Input: part model. Units: mm. Frame: model coordinates. Coordinates: 2 decimals unless noted, no trailing zeros. Write each loop counter-clockwise with the first axis right and the second up, starting at its lowest first coordinate (ties: lowest second). Pieces come first, ordered by that corner, then holes. Notation, with made-up numbers: (40, 19.25) -> (52, 19.25) arc R27 ccw to (52, 43.25) -> close; hole circle Ø2 at (89, 51.25). An arc over 180 degrees is marked (long way). Use one line per item in the form item = value. Start each with the question number.
(1) Cut plane D-D on x = 15.5. Return the cut outline in (y, z), plus the area to 3 significant figures.
(2) Ray query, line 1 along Z through (x, y) = (-4, 0.9); line 2 along Z through (x, y) = (0, 0.5); line 3 along X through (y, z) = (1, 1.75). Return the intervals inside material, ascending.
(3) Cut plane A-A on y = 1. State how many separate pieces and enclosed holes the cut face has, plus the area to 3 significant figures.
(4) First-contact query: pin 1 (4 mm diameter, centred on x = 16, z = 1.5, fed in from -Y). Flat tip, straight axial feed; report the tip coordinate or a pass-through.
(5) Cut plane C-C on x = -8. Return the cut outline in (y, z), plus the area to 3 significant figures.
(6) Cut plane B-B on x = 3. Return the cut outline in (y, z), plus the area to 3 significant figures.
Autodesk Inventor part; units mm, degrees
ref_plane "YZ Plane" through (0, 0, 0) normal (1, 0, 0) x (0, 1, 0)
ref_plane "XZ Plane" through (0, 0, 0) normal (0, 1, 0) x (-1, 0, 0)
ref_plane "XY Plane" through (0, 0, 0) normal (0, 0, 1) x (1, 0, 0)
sketch "Sketch2" plane through (0, 0, 0) normal (0, 1, 0) x (-1, 0, 0)
  line L0 (-32, 4) -> (32, 4)
  line L1 (32, 4) -> (32, -4)
  line L2 (32, -4) -> (-32, -4)
  line L3 (-32, -4) -> (-32, 4)
  point P0 (0, 0)
  point P1 (0, 4)
  point P2 (-32, 0)
  dimension "d0" = 64
  dimension "d1" = 8
extrude "Extrusion1" add sketch "Sketch2" along normal blind 3.2
sketch "Sketch3" plane through (0, 0, 0) normal (0, -1, 0) x (1, 0, 0)
  line L0 (32, 4) -> (-32, 4)
  line L1 (-32, 4) -> (-32, -4)
  line L2 (-30.4, 2.4) -> (30.4, 2.4)
  line L3 (30.4, 2.4) -> (30.4, -2.4)
  line L4 (30.4, -2.4) -> (-30.4, -2.4)
  line L5 (-30.4, -2.4) -> (-30.4, 2.4)
  circle A0 centre (-24, 4) radius 3.2569
  circle A1 centre (-24, 4) radius 2.4
  line L6 (-32, -4) -> (32, -4)
  circle A2 centre (0, 0) radius 1.6
  line L7 (32, -4) -> (32, 4)
  line L8 (-20, 0) -> (-12, 0) construction
  line L9 (-12, 0) -> (-4, 0) construction
  line L10 (4, 0) -> (12, 0) construction
  line L11 (12, 0) -> (20, 0) construction
  line L12 (-4, 0) -> (4, 0) construction
  line L13 (-28, 0) -> (-20, 0) construction
  line L14 (20, 0) -> (28, 0) construction
  line L15 (-31.6, 3.6) -> (31.6, 3.6)
  line L16 (31.6, 3.6) -> (31.6, -3.6)
  line L17 (31.6, -3.6) -> (-31.6, -3.6)
  line L18 (-31.6, -3.6) -> (-31.6, 3.6)
  point P0 (-30.4, 0)
  point P1 (0, 2.4)
  point P2 (0, 3.6)
  point P3 (-31.6, 0)
  dimension "d8" = 1.6
  dimension "d60" = 6.5137
  dimension "d61" = 4.8
  dimension "d62" = 1.6
  dimension "d75" = 8
  dimension "d76" = 8
  dimension "d86" = 3.2
  dimension "d93" = 8
  dimension "d99" = 0.4
  dimension "d100" = 0.4
extrude "Extrusion2" cut sketch "Sketch3" against normal blind 1.6 contours A0 L2 A1 | L2 L3 L4 L5 A0 | A1 L2 | A2
extrude "Extrusion7" cut sketch "Sketch3" against normal blind 0.4 contours L7 L6 L1 L0 A0 L15 L18 L17 L16 | A0 L15 A1 L0 | A1 L15 L0 | L0 A1 L15 A0
extrude "Extrusion6" add sketch "Sketch3" against normal up to next contours A2
pattern_linear "Rectangular Pattern3" count 7 spacing 8 along (-1, 0, 0) of "Extrusion6" first direction both ways yes
fillet "Fillet1" radius 0.1 8 edges at (-32, 1.8, 4) (0, 3.2, 4) (-32, 3.2, 0) (32, 1.8, 4) (32, 3.2, 0) (0, 3.2, -4) (32, 1.8, -4) (-32, 1.8, -4)
equation "\"d4\" = 0.333333 * lh"
equation "\"d8\" = d62"
equation "\"d60\" = tubeod"
equation "\"d61\" = kd"
equation "\"d62\" = wall"
equation "\"d75\" = lu"
equation "\"d76\" = d75"
equation "\"d86\" = pd"
equation "\"d93\" = lu"
equation "\"d99\" = gw"
equation "\"d100\" = gw"
equation "\"d11\" = 0.333333 * lh - topthk"
equation "\"d101\" = gh"
equation "\"d91\" = lu"
equation "\"d22\" = lf"
properties part number "4162-LtBluishGray" material "ABS Plastic"
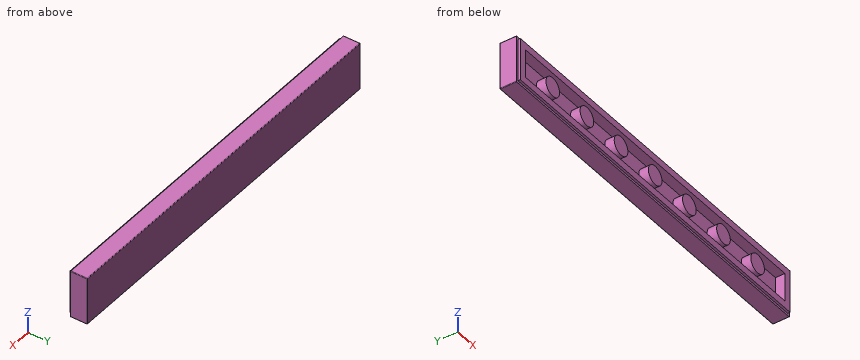
Values:
q1.outline = (0, -3.6) -> (0.4, -3.6) -> (0.4, -4) -> (3.1, -4) arc R0.1 ccw to (3.2, -3.9) -> (3.2, 3.9) arc R0.1 ccw to (3.1, 4) -> (0.4, 4) -> (0.4, 3.6) -> (0, 3.6) -> (0, 2.4) -> (1.6, 2.4) -> (1.6, 1.52) -> (0, 1.52) -> (0, -1.52) -> (1.6, -1.52) -> (1.6, -2.4) -> (0, -2.4) -> close
q1.area = 22.5 mm2
q2.line_1 = -4 to -2.4, 2.4 to 4
q2.line_2 = -4 to -2.4, -1.6 to 1.6, 2.4 to 4
q2.line_3 = -32 to -30.4, 30.4 to 32
q3.separate_pieces = 8
q3.enclosed_holes = 1
q3.area = 276 mm2
q4.pin_1 = 0
q5.outline = (0, -3.6) -> (0.4, -3.6) -> (0.4, -4) -> (3.1, -4) arc R0.1 ccw to (3.2, -3.9) -> (3.2, 3.9) arc R0.1 ccw to (3.1, 4) -> (0.4, 4) -> (0.4, 3.6) -> (0, 3.6) -> (0, 2.4) -> (1.6, 2.4) -> (1.6, 1.6) -> (0, 1.6) -> (0, -1.6) -> (1.6, -1.6) -> (1.6, -2.4) -> (0, -2.4) -> close
q5.area = 22.7 mm2
q6.outline = (0, -3.6) -> (0.4, -3.6) -> (0.4, -4) -> (3.1, -4) arc R0.1 ccw to (3.2, -3.9) -> (3.2, 3.9) arc R0.1 ccw to (3.1, 4) -> (0.4, 4) -> (0.4, 3.6) -> (0, 3.6) -> (0, 2.4) -> (1.6, 2.4) -> (1.6, -2.4) -> (0, -2.4) -> close
q6.area = 17.6 mm2
